from build123d import *

# Parameters (mm, degrees)
F0_W         = 152.4
F0_H         = 152.4
F1_DEPTH     = 76.2
F2_R         = 12.8651099241
F2_R_2       = 12.0389782125
F2_R_3       = 13.4461105648
F2_R_4       = 11.9959461494
F3_DEPTH     = 25.4
F4_T         = 2.54
F5_T1_DEPTH  = 147.32
F5_T3_DEPTH  = 147.32
F5_T9_DEPTH  = 160.02
F5_T15_DEPTH = 160.02
F5_T24_DEPTH = 160.02
F5_T30_DEPTH = 160.02
F5_T39_DEPTH = 160.02
F5_T45_DEPTH = 160.02
F5_T54_DEPTH = 160.02
F5_T60_DEPTH = 160.02
F6_W         = 16.6622009128
F6_H         = 28.2943053171
F6_H_2       = 16.9765818864
F6_W_2       = 27.9799224809
F7_DEPTH     = 25.4
F8_R         = 5.4524649891
F8_R_2       = 5.9328095345
F8_R_3       = 6.7719768786
F8_R_4       = 7.5712998573
F9_DEPTH     = 25.4
F11_DEPTH    = 25.4


# Not quite as in the source:
# - a fillet or chamfer that OpenCascade refuses, or shapes differently, is made with other operations: its cross-section is extruded or revolved along the edge and cut away or added
# - a shell that OpenCascade refuses in one call is made with other operations: the cavity is built on its own and cut out


with BuildPart() as f1:
    # F0 (on Front) → F1 (new body)
    with BuildSketch(Plane.XZ):
        Rectangle(F0_W, F0_H)
    extrude(amount=F1_DEPTH)

    # F2 (on face) → F3 (cut)
    with BuildSketch(Plane.XZ):
        with Locations((57.6343238354, 59.4989620149)):
            Circle(F2_R)
        with Locations((-57.2953000665, 60.177013278)):
            Circle(F2_R_2)
        with Locations((58.6513988674, -59.8379895091)):
            Circle(F2_R_3)
        with Locations((-60.6855526567, -60.8550645411)):
            Circle(F2_R_4)
    extrude(amount=F3_DEPTH, mode=Mode.SUBTRACT)

    # F4: shell of thickness 2.54, made by hand


with BuildPart() as f4_core1:
    # F4_t2: copy of F1
    add(f1.part)

    # the walls: a layer under each face that stays
    f4_faces = [f4_core1.faces().sort_by_distance(p)[0] for p in [
        (0, -38.1, 76.2),
        (76.2, -38.1, 0),
        (-76.2, -38.1, 0),
        (0, 0, 0),
        (0, -38.1, -76.2),
        (-72.681498806, -12.7, -60.8550645411),
        (45.2052883026, -12.7, -59.8379895091),
        (-69.334278279, -12.7, 60.177013278),
        (44.7692139113, -12.7, 59.4989620149),
        (-60.6855526567, -25.4, -60.8550645411),
        (58.6513988674, -25.4, -59.8379895091),
        (-57.2953000665, -25.4, 60.177013278),
        (57.6343238354, -25.4, 59.4989620149),
    ]]
    thicken(f4_faces, amount=-F4_T, mode=Mode.SUBTRACT)

    # F4_s3 → F4_t4 (revolve, cut)
    with BuildSketch(Plane.XY.offset(-60.8550645411)):
        Polygon((-48.7150065073, -25.3746), (-46.1496065073, -25.4), (-46.1496065073, -27.94), (-48.6896065073, -27.94), align=None)
    revolve(axis=Axis((-60.6855526567, -25.4, -60.8550645411), (0, -1, 0)), mode=Mode.SUBTRACT)

    # F4_s5 → F4_t6 (revolve, cut)
    with BuildSketch(Plane.XY.offset(-59.8379895091)):
        Polygon((72.0721094321, -25.3746), (74.6375094321, -25.4), (74.6375094321, -27.94), (72.0975094321, -27.94), align=None)
    revolve(axis=Axis((58.6513988674, -25.4, -59.8379895091), (0, -1, 0)), mode=Mode.SUBTRACT)

    # F4_s7 → F4_t8 (revolve, cut)
    with BuildSketch(Plane.XY.offset(60.177013278)):
        Polygon((-45.281721854, -25.3746), (-42.716321854, -25.4), (-42.716321854, -27.94), (-45.256321854, -27.94), align=None)
    revolve(axis=Axis((-57.2953000665, -25.4, 60.177013278), (0, -1, 0)), mode=Mode.SUBTRACT)

    # F4_s9 → F4_t10 (revolve, cut)
    with BuildSketch(Plane.XY.offset(59.4989620149)):
        Polygon((70.4740337595, -25.3746), (73.0394337595, -25.4), (73.0394337595, -27.94), (70.4994337595, -27.94), align=None)
    revolve(axis=Axis((57.6343238354, -25.4, 59.4989620149), (0, -1, 0)), mode=Mode.SUBTRACT)


with BuildPart() as f1_1:
    add(f1.part)

    # what is left inside the walls is the cavity
    f4_cavity = [f4_core1.part.solids().sort_by_distance(p)[0] for p in [
        (0, -76.1746, -24.553333),
    ]]
    add(f4_cavity, mode=Mode.SUBTRACT)

    # F5: fillet of radius 5.08 on 4 edges, made by hand

    # F5_s2 → F5_t1 (cut)
    with BuildSketch(Plane.YZ.offset(-73.66)):
        with BuildLine():
            ThreePointArc((-76.2, 78.74), (-74.7121024484, 75.1478975516), (-71.12, 73.66))
            Line((-71.12, 73.66), (-76.2, 73.66))
            Line((-76.2, 73.66), (-76.2, 78.74))
        make_face()
        with BuildLine():
            ThreePointArc((-76.2, -78.74), (-74.7121024484, -75.1478975516), (-71.12, -73.66))
            Line((-71.12, -73.66), (-76.2, -73.66))
            Line((-76.2, -73.66), (-76.2, -78.74))
        make_face()
    extrude(amount=F5_T1_DEPTH, mode=Mode.SUBTRACT)

    # F5_s4 → F5_t3 (cut)
    with BuildSketch(Plane.XY.offset(-73.66)):
        with BuildLine():
            ThreePointArc((-78.74, -76.2), (-75.1478975516, -74.7121024484), (-73.66, -71.12))
            Line((-73.66, -71.12), (-73.66, -76.2))
            Line((-73.66, -76.2), (-78.74, -76.2))
        make_face()
        with BuildLine():
            ThreePointArc((78.74, -76.2), (75.1478975516, -74.7121024484), (73.66, -71.12))
            Line((73.66, -71.12), (73.66, -76.2))
            Line((73.66, -76.2), (78.74, -76.2))
        make_face()
    extrude(amount=F5_T3_DEPTH, mode=Mode.SUBTRACT)


with BuildPart() as f5_tool7:
    # F5_s8 → F5_t9 (new body)
    with BuildSketch(Plane.YZ.offset(86.36)):
        with BuildLine():
            ThreePointArc((-76.2, 78.74), (-74.7121024484, 75.1478975516), (-71.12, 73.66))
            Line((-71.12, 73.66), (-76.2, 73.66))
            Line((-76.2, 73.66), (-76.2, 78.74))
        make_face()
    extrude(amount=-F5_T9_DEPTH)

    split(bisect_by=Plane.XY.offset(76.2), keep=Keep.BOTTOM)

    split(bisect_by=Plane.YZ.offset(76.2), keep=Keep.BOTTOM)

    split(bisect_by=Plane.YZ.offset(73.66), keep=Keep.TOP)


with BuildPart() as f5_tool13:
    # F5_s14 → F5_t15 (new body)
    with BuildSketch(Plane.XY.offset(-73.66)):
        with BuildLine():
            ThreePointArc((78.74, -76.2), (75.1478975516, -74.7121024484), (73.66, -71.12))
            Line((73.66, -71.12), (73.66, -76.2))
            Line((73.66, -76.2), (78.74, -76.2))
        make_face()
    extrude(amount=F5_T15_DEPTH)

    split(bisect_by=Plane.XY.offset(76.2), keep=Keep.BOTTOM)

    split(bisect_by=Plane.YZ.offset(76.2), keep=Keep.BOTTOM)

    split(bisect_by=Plane.XY.offset(73.66), keep=Keep.TOP)


with BuildPart() as f5_tool7_1:
    add(f5_tool7.part)

    # F5_t19: intersect F5_tool13
    add(f5_tool13.part, mode=Mode.INTERSECT)


with BuildPart() as f1_2:
    add(f1_1.part)

    # F5_t5: cut F5_tool7
    add(f5_tool7_1.part, mode=Mode.SUBTRACT)


with BuildPart() as f5_tool22:
    # F5_s23 → F5_t24 (new body)
    with BuildSketch(Plane.YZ.offset(73.66)):
        with BuildLine():
            ThreePointArc((-76.2, 78.74), (-74.7121024484, 75.1478975516), (-71.12, 73.66))
            Line((-71.12, 73.66), (-76.2, 73.66))
            Line((-76.2, 73.66), (-76.2, 78.74))
        make_face()
    extrude(amount=-F5_T24_DEPTH)

    split(bisect_by=Plane.XY.offset(76.2), keep=Keep.BOTTOM)

    split(bisect_by=Plane.YZ.offset(-76.2), keep=Keep.TOP)

    split(bisect_by=Plane.YZ.offset(-73.66), keep=Keep.BOTTOM)


with BuildPart() as f5_tool28:
    # F5_s29 → F5_t30 (new body)
    with BuildSketch(Plane.XY.offset(86.36)):
        with BuildLine():
            ThreePointArc((-78.74, -76.2), (-75.1478975516, -74.7121024484), (-73.66, -71.12))
            Line((-73.66, -71.12), (-73.66, -76.2))
            Line((-73.66, -76.2), (-78.74, -76.2))
        make_face()
    extrude(amount=-F5_T30_DEPTH)

    split(bisect_by=Plane.XY.offset(76.2), keep=Keep.BOTTOM)

    split(bisect_by=Plane.YZ.offset(-76.2), keep=Keep.TOP)

    split(bisect_by=Plane.XY.offset(73.66), keep=Keep.TOP)


with BuildPart() as f5_tool22_1:
    add(f5_tool22.part)

    # F5_t34: intersect F5_tool28
    add(f5_tool28.part, mode=Mode.INTERSECT)


with BuildPart() as f1_3:
    add(f1_2.part)

    # F5_t20: cut F5_tool22
    add(f5_tool22_1.part, mode=Mode.SUBTRACT)


with BuildPart() as f5_tool37:
    # F5_s38 → F5_t39 (new body)
    with BuildSketch(Plane.XY.offset(73.66)):
        with BuildLine():
            ThreePointArc((-78.74, -76.2), (-75.1478975516, -74.7121024484), (-73.66, -71.12))
            Line((-73.66, -71.12), (-73.66, -76.2))
            Line((-73.66, -76.2), (-78.74, -76.2))
        make_face()
    extrude(amount=-F5_T39_DEPTH)

    split(bisect_by=Plane.YZ.offset(-76.2), keep=Keep.TOP)

    split(bisect_by=Plane.XY.offset(-76.2), keep=Keep.TOP)

    split(bisect_by=Plane.XY.offset(-73.66), keep=Keep.BOTTOM)


with BuildPart() as f5_tool43:
    # F5_s44 → F5_t45 (new body)
    with BuildSketch(Plane.YZ.offset(-86.36)):
        with BuildLine():
            ThreePointArc((-76.2, -78.74), (-74.7121024484, -75.1478975516), (-71.12, -73.66))
            Line((-71.12, -73.66), (-76.2, -73.66))
            Line((-76.2, -73.66), (-76.2, -78.74))
        make_face()
    extrude(amount=F5_T45_DEPTH)

    split(bisect_by=Plane.YZ.offset(-76.2), keep=Keep.TOP)

    split(bisect_by=Plane.XY.offset(-76.2), keep=Keep.TOP)

    split(bisect_by=Plane.YZ.offset(-73.66), keep=Keep.BOTTOM)


with BuildPart() as f5_tool37_1:
    add(f5_tool37.part)

    # F5_t49: intersect F5_tool43
    add(f5_tool43.part, mode=Mode.INTERSECT)


with BuildPart() as f1_4:
    add(f1_3.part)

    # F5_t35: cut F5_tool37
    add(f5_tool37_1.part, mode=Mode.SUBTRACT)


with BuildPart() as f5_tool52:
    # F5_s53 → F5_t54 (new body)
    with BuildSketch(Plane.YZ.offset(-73.66)):
        with BuildLine():
            ThreePointArc((-76.2, -78.74), (-74.7121024484, -75.1478975516), (-71.12, -73.66))
            Line((-71.12, -73.66), (-76.2, -73.66))
            Line((-76.2, -73.66), (-76.2, -78.74))
        make_face()
    extrude(amount=F5_T54_DEPTH)

    split(bisect_by=Plane.YZ.offset(76.2), keep=Keep.BOTTOM)

    split(bisect_by=Plane.XY.offset(-76.2), keep=Keep.TOP)

    split(bisect_by=Plane.YZ.offset(73.66), keep=Keep.TOP)


with BuildPart() as f5_tool58:
    # F5_s59 → F5_t60 (new body)
    with BuildSketch(Plane.XY.offset(-86.36)):
        with BuildLine():
            ThreePointArc((78.74, -76.2), (75.1478975516, -74.7121024484), (73.66, -71.12))
            Line((73.66, -71.12), (73.66, -76.2))
            Line((73.66, -76.2), (78.74, -76.2))
        make_face()
    extrude(amount=F5_T60_DEPTH)

    split(bisect_by=Plane.YZ.offset(76.2), keep=Keep.BOTTOM)

    split(bisect_by=Plane.XY.offset(-76.2), keep=Keep.TOP)

    split(bisect_by=Plane.XY.offset(-73.66), keep=Keep.BOTTOM)


with BuildPart() as f5_tool52_1:
    add(f5_tool52.part)

    # F5_t64: intersect F5_tool58
    add(f5_tool58.part, mode=Mode.INTERSECT)


with BuildPart() as f1_5:
    add(f1_4.part)

    # F5_t50: cut F5_tool52
    add(f5_tool52_1.part, mode=Mode.SUBTRACT)

    # F6 (on face) → F7 (cut)
    with BuildSketch(Plane.XZ.offset(2.54)):
        with Locations((0, 22.6354436018)):
            Rectangle(F6_W, F6_H)
        Rectangle(F6_W, F6_H_2)
        with Locations((0, -22.6354436018)):
            Rectangle(F6_W, F6_H)
        with Locations((22.3210616969, 0)):
            Rectangle(F6_W_2, F6_H_2)
        with Locations((-22.3210616969, 0)):
            Rectangle(F6_W_2, F6_H_2)
    extrude(amount=-F7_DEPTH, mode=Mode.SUBTRACT)

    # F8 (on face) → F9 (cut)
    with BuildSketch(Plane.XZ.offset(27.94)):
        with Locations((-62.8410799733, -61.9330853224)):
            Circle(F8_R)
        with Locations((-57.2953000665, 60.177013278)):
            Circle(F8_R_2)
        with Locations((56.4314164221, 60.6755614281)):
            Circle(F8_R_3)
        with Locations((58.3177022636, -59.4180375338)):
            Circle(F8_R_4)
    extrude(amount=-F9_DEPTH, mode=Mode.SUBTRACT)

    # F10 (on face) → F11 (cut)
    with BuildSketch(Plane.XZ):
        Polygon((17.9349766593, -45.055488267), (30.337780714, -50.615362823), (38.728027374, -30.3751360907), (52.3444600403, 0), (31.5953046083, 21.0635364056), (41.6555032134, 3.458192572), (36.6254039109, -21.6922983527), align=None)
        Polygon((-30.652159825, -50.3551833958), (-26.879588142, -37.4113582075), (-44.5359825398, -29.4964272347), (-44.5359825398, -9.7458148375), (-62.0902739465, 5.9732417576), (-65.8628493547, 24.8361118138), (-70.892944932, 3.458192572), (-53.9163686335, -14.7759132087), (-53.9163686335, -39.9264059961), align=None)
        Polygon((-42.5986461341, 40.5551679432), (-30.652159825, 35.5250686407), (-24.3645366281, 49.3578389287), (-24.3645366281, 59.4180375338), (-13.6755788699, 71.3645219803), (-31.9096893072, 63.8193711638), (-31.9096893072, 51.8728867173), align=None)
        Polygon((32.2240665555, 31.7524932325), (38.9561592304, 39.308484465), (34.110352397, 50.615362823), (20.2775839716, 50.615362823), (13.3611978963, 63.1906092167), (0, 66.334426403), (7.7023385093, 53.1304106116), (25.9364452213, 44.9565052986), align=None)
    extrude(amount=F11_DEPTH, mode=Mode.SUBTRACT)


solid = f1_5.part
Could you check a few things on this model? Use its own coordinates, in mm. A direction names the side the tool comes from. Coordinates: 2 decimals unless noted, no trailing zeros. Order: outer loops, then holes, each group sorted by start corner. A loop starts at its lowest first (then second) coordinate and runs counter-clockwise, first axis right, second up. Notation, with made-up numbers: (-25, 73.25) - (-6, 73.25) arc R21 cw to (-6, 100.25) - close; hole circle Ø8 at (-29, -27.5). An arc over 180 degrees is marked (long way). Answer in a Markdown table with one row per item. Add a question column.
(1) On a 3-axis mill with a long thin cutter (end or side, diameter ignored), from which of +Z, -Z, +X, -X, +Y, -Y can I reach the whole of each face in a straight line? I mean faces 1 (the face through (-1.07, -73.69, -74.36)), 2 (the face through (48.74, -12.52, -50.75)), 3 (the face through (16.87, -1.25, 56.81)). Say none if no direction works.
(2) If we section it at C-C, the plane x = -40: Please give me the cut outline in (y, z).
(3) Will this pin go through, and if not, where does the flat tip stop? pin 1 (6 mm diameter, centred on x = -13.5, z = 54, fed in from -Y).
(4) If we section it at A-A, the plane z = 13.5: Please give me the cut outline in (x, y), then the cut area to 3 significant figures.
(5) I need wall thicknesses on L1, parallel to Z at x = -19, y = -38.5; L2, parallel to X at y = -26.5, z = 55. Which ranges of each line are inside material? Lowest first, please.
(6) If we section it at D-D, the plane y = -21.5: Please give me the cut outline in (x, z), then the cut area to 3 significant figures.
(7) If we section it at B-B, the plane y = -49: Please give me the cut outline in (x, z), then the cut area to 3 significant figures.
Results are:
| question | item | result |
|---|---|---|
| 1 | face 1 | -Y |
| 1 | face 2 | +Y |
| 1 | face 3 | +Y, -Y |
| 2 | outline | (-75.52, -76.2) - (0, -76.2) - (0, -46.16) - (-2.54, -46.16) - (-2.54, -73.66) - (-71.12, -73.66) arc R5.08 ccw to start; (-75.52, 76.2) arc R5.08 ccw to (-71.12, 73.66) - (-2.54, 73.66) - (-2.54, 43.31) - (0, 43.31) - (0, 76.2) - close; (-2.54, -31.53) - (0, -31.53) - (0, 39.46) - (-2.54, 39.46) - close |
| 3 | pin 1 | stops at y = -2.54 |
| 4 | outline | (-76.2, -75.52) arc R5.08 ccw to (-73.66, -71.12) - (-73.66, -2.54) - (-68.53, -2.54) - (-68.53, 0) - (-76.2, 0) - close; (-63.6, -2.54) - (-8.33, -2.54) - (-8.33, 0) - (-63.6, 0) - close; (8.33, -2.54) - (35.92, -2.54) - (35.92, 0) - (8.33, 0) - close; (39.05, -2.54) - (73.66, -2.54) - (73.66, -71.12) arc R5.08 ccw to (76.2, -75.52) - (76.2, 0) - (39.05, 0) - close |
| 4 | area | 689 mm2 |
| 5 | L1 | z = -76.2 to -73.66, 73.66 to 76.2 |
| 5 | L2 | x = -76.2 to -73.66, -70.92 to -60.19, -54.4 to -43.67, 42.9 to 52.74, 60.13 to 72.37, 73.66 to 76.2 |
| 6 | outline | (-76.2, -76.2) - (76.2, -76.2) - (76.2, 76.2) - (-76.2, 76.2) - close; hole (-73.66, -73.66) - (-67.57, -73.66) arc R14.54 cw to (-73.66, -67.41) - close; hole (-73.66, -54.3) arc R14.54 cw (long way) to (-53.81, -73.66) - (50.62, -73.66) arc R15.99 cw (long way) to (73.66, -54.33) - (73.66, 73.66) - (63.7, 73.66) arc R15.41 cw (long way) to (51.57, 73.66) - (-51.75, 73.66) arc R14.58 cw (long way) to (-62.84, 73.66) - (-73.66, 73.66) - close; hole circle Ø23.99 at (-60.69, -60.86); hole circle Ø24.08 at (-57.3, 60.18); hole circle Ø25.73 at (57.63, 59.5); hole circle Ø26.89 at (58.65, -59.84); hole (66.68, -73.66) - (73.66, -73.66) - (73.66, -65.34) arc R15.99 cw to start |
| 6 | area | 2,330 mm2 |
| 7 | outline | (-76.2, -76.2) - (76.2, -76.2) - (76.2, 76.2) - (-76.2, 76.2) - close; hole (-73.66, -73.66) - (73.66, -73.66) - (73.66, 73.66) - (-73.66, 73.66) - close |
| 7 | area | 1,520 mm2 |
